Check sheet for the drawn part. Datum: minimum x, y, z corner. Units: mm. Coordinates: 2 decimals unless noted, no trailing zeros. Order: outer loops, then holes, each group sorted by start corner. A loop starts at its lowest first (then second) coordinate and runs counter-clockwise, first axis right, second up. Notation, with made-up numbers: (77, -13) - (102, -13) arc R6 cw to (102, -9) - close; hole circle Ø5 at (-22.75, -27). An arc over 180 degrees is marked (long way). Put each result on its own line as item: value.
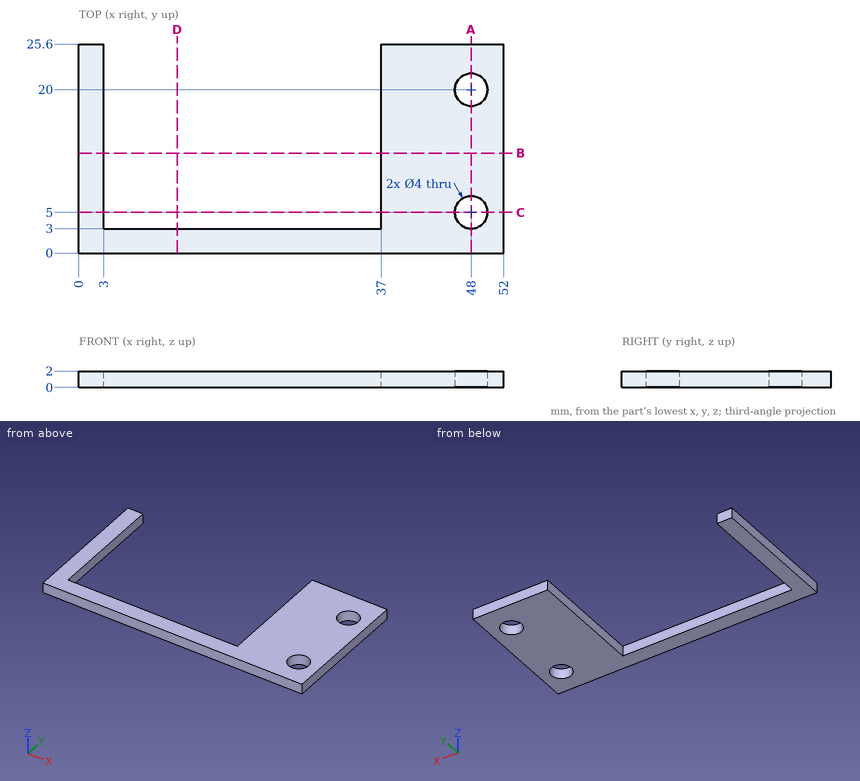
Q1. Section check D-D on x = 12. Record the boundary of the cut face in (y, z).
Answer block:
outline: (0, 0) - (3, 0) - (3, 2) - (0, 2) - close
Q2. Depth check by flat-ended pin: pin 1 Ø0.6 at (x, z) = (12, 1.5) entering from +Y. Enter the tip coordinate at first touch or a pass-through.
Answer block:
pin 1: stops at y = 3
Q3. Section check C-C on y = 5. Record the boundary of the cut face in (x, z).
Answer block:
outline: (0, 0) - (3, 0) - (3, 2) - (0, 2) - close; (37, 0) - (46, 0) - (46, 2) - (37, 2) - close; (50, 0) - (52, 0) - (52, 2) - (50, 2) - close
Q4. Section check B-B on y = 12.25. Record the boundary of the cut face in (x, z), then the cut area to 3 significant figures.
Answer block:
outline: (0, 0) - (3, 0) - (3, 2) - (0, 2) - close; (37, 0) - (52, 0) - (52, 2) - (37, 2) - close
area: 36.0 mm^2
Q5. Thickness scan on L1, parallel to Y at x = 48, z = 1.05; L2, parallel to X at y = 5, z = 0.95; L3, parallel to X at y = 16.75, z = 1.7. Record the ranges inside material, lowest first. Write a range as [from, to].
Answer block:
L1: y = [0, 3], [7, 18], [22, 25.6]
L2: x = [0, 3], [37, 46], [50, 52]
L3: x = [0, 3], [37, 52]
Q6. Section check A-A on x = 48. Record the boundary of the cut face in (y, z).
Answer block:
outline: (0, 0) - (3, 0) - (3, 2) - (0, 2) - close; (7, 0) - (18, 0) - (18, 2) - (7, 2) - close; (22, 0) - (25.6, 0) - (25.6, 2) - (22, 2) - close
